CAD build for the part. Positions are in the model's coordinates, mm. A direction names the side the tool comes from. Coordinates: 2 decimals unless noted, no trailing zeros. Order: outer loops, then holes, each group sorted by start corner. A loop starts at its lowest first (then second) coordinate and runs counter-clockwise, first axis right, second up. Notation, with made-up numbers: M 36.25,-32.75 L 56.25,-32.75 A6 ccw 56.25,-23.75 Z; hole C 35,21 d3. An arc over 180 degrees is marked long. One line per item, written item: value.
from build123d import *

# Parameters (mm, degrees)
SKETCH2_W          = 94.742
SKETCH2_H          = 28.575
BASE_FLANGE1_DEPTH = 3.175
EDGE_FLANGE1_DEPTH = 28.575
CUT_EXTRUDE2_DEPTH = 3.175


# Sheet-metal steps are written as plain solids
with BuildPart() as part:
    # Sketch2 → Base-Flange1 (new body)
    with BuildSketch(Plane.XY):
        Rectangle(SKETCH2_W, SKETCH2_H)
    extrude(amount=BASE_FLANGE1_DEPTH)

    # Edge-Flange1 section (across the edge) → Edge-Flange1 (add)
    with BuildSketch(Plane(origin=(48.371, -14.2875, 3.175), x_dir=(-1, 0, 0), z_dir=(0, 1, 0))):
        with BuildLine():
            Line((-3.175, 1), (-3.175, 41.275))
            Line((-3.175, 41.275), (0, 41.275))
            Line((0, 41.275), (0, 1))
            ThreePointArc((0, 1), (0.292893219, 0.292893219), (1, 0))
            Line((1, 0), (1, -3.175))
            ThreePointArc((1, -3.175), (-1.952170811, -1.952170811), (-3.175, 1))
        make_face()
    extrude(amount=EDGE_FLANGE1_DEPTH)

    # Sketch11 → Cut-Extrude2 (cut)
    with BuildSketch(Plane(origin=(51.546, 0, 0), x_dir=(0, 0, -1), z_dir=(1, 0, 0))):
        Polygon((-44.45, -14.2875), (-4.175, 14.2875), (-44.45, 14.2875), align=None)
    extrude(amount=-CUT_EXTRUDE2_DEPTH, mode=Mode.SUBTRACT)


solid = part.part
Q1. Slice it at D-D (y = -3.75). List the corners of the cut face in (x, z) (3 decimals).
Recorded:
outline: M -47.371,0 L 47.371,0 A4.175 ccw 51.546,4.175 L 51.546,29.598 L 48.371,29.598 L 48.371,4.175 A1 cw 47.371,3.175 L -47.371,3.175 Z
Q2. Slice it at B-B (x = 14). List the corners of the cut face in (y, z) (1 decimal).
Recorded:
outline: M -14.3,0 L 14.3,0 L 14.3,3.2 L -14.3,3.2 Z
Q3. Slice it at A-A (y = -10.5). List the corners of the cut face in (x, z) (3 decimals), plus the area to 3 significant figures.
Recorded:
outline: M -47.371,0 L 47.371,0 A4.175 ccw 51.546,4.175 L 51.546,39.112 L 48.371,39.112 L 48.371,4.175 A1 cw 47.371,3.175 L -47.371,3.175 Z
area: 425 mm^2
Q4. Drill centre lines: line 1 along Z through (x, y) = (1, -12.75) (3 decimals); line 2 along X through (y, z) = (2.5, 12); line 3 along X through (y, z) = (-10.75, 3.5). Where is each one in solid material? Low to high.
Recorded:
line 1: z = 0 to 3.175
line 2: x = 48.37 to 51.55
line 3: x = 48.11 to 51.49
Q5. Slice it at C-C (z = 38). List the corners of the cut face in (x, y).
Recorded:
outline: M 48.37,-14.29 L 51.55,-14.29 L 51.55,-9.71 L 48.37,-9.71 Z
Q6. Pin check, flat tips, straight feed: pin 1 Ø12 at (x, y) = (20.5, -10) entering from +Z (3 decimals); pin 2 Ø6 at (y, z) = (-5.5, 20.5) entering from -X. Stop position of each tip, or through.
Recorded:
pin 1: stops at z = 3.175
pin 2: stops at x = 48.37
Q7. Which spindle directions (+Z, -Z, +X, -X, +Y, -Y) get a long thin tool onto all of the face, cutting with end or side? Do faces 1 (the face through (48.371, -7, 16)), 2 (the face through (-1, 0, 0)). Say none if no direction does.
Recorded:
face 1: +Z, -X, +Y, -Y
face 2: -Z, +X, -X, +Y, -Y
